Geometry: final body of the model. Coordinates: model frame, mm. A direction names the side the tool comes from. Round coordinates to 2 decimals unless told otherwise and drop trailing zeros. Write each loop counter-clockwise with the first axis right and the second up, starting at its lowest first coordinate (ties: lowest second). Pieces come first, ordered by that corner, then holes. Notation, with made-up numbers: M 52.5,-19.75 L 85.5,-19.75 A21 ccw 85.5,-8.75 Z; hole C 42,31.5 d6. An arc over 180 degrees is marked long. Answer as CSV lines item,"result". Start each with the question number.
Q1. First-contact query: pin 1 (4 mm diameter, centred on y = 25, z = -8, fed in from -X); pin 2 (19.5 mm diameter, centred on x = 14, y = 10, fed in from -Z); pin 3 (19.5 mm diameter, centred on x = 5.5, y = 25.5, fed in from +Z). Flat tips, straight axial feed; report the tip coordinate or a pass-through.
Q2. Ray query, probe 1 along Z at (x, y) = (24, 19.5); probe 2 along X at (y, z) = (25, 31.5); probe 3 along Z at (x, y) = (23.5, 29.5). Return the intervals inside material, ascending.
Q3. Section query D-D on y = 33.5. Output: boundary loops of the cut face in (x, z).
Q4. Section query B-B on z = 17. Output: boundary loops of the cut face in (x, y).
Q5. Section query C-C on x = 0. Output: boundary loops of the cut face in (y, z).
Q6. Mould query, pull axis X, two halves, no side actions, for faces 1 (the flat face through (0, 0, 9)), 2 (the cylindrical face through (5.5, 17.77, -9.87)), 3 (the flat face through (0, 19, 9.206)). Classes: pulls with the +X half, pulls with the -X half, needs draft (parallel to the pull), parting line crosses it, or undercut.
Q7. Reachability of faces 4 (the flat face through (20.554, 19, 20)), 5 (the flat face through (-30.313, 19, 17)) from +Z, -Z, +X, -X, +Y, -Y: full face, straight path, thin tool, end or side. Return the list, or none.
Q8. Section query A-A on y = 19.5. Output: boundary loops of the cut face in (x, z), and give its area (3 significant figures).
```python
from build123d import *

# Parameters (mm, degrees)
F1_DEPTH = 39
F3_R     = 5.308104
F4_DEPTH = 60.626907
F5_R     = 5.76541
F6_DEPTH = 14.8


with BuildPart() as f1:
    # F0 (on Front) → F1 (new body)
    with BuildSketch(Plane.XZ):
        Polygon((0, 9.205531), (0, -2.570523), (30.312954, -2.570523), (30.312954, 36.376152), (20.553786, 36.376152), (20.553786, 9.205531), align=None)
    extrude(amount=-F1_DEPTH)

    # F2: F1 across face


with BuildPart() as f1_1:
    add(f1.part)
    add(f1.part.mirror(Plane(origin=(0, 19.5, 3.317504), x_dir=(0, -1, 0), z_dir=(-1, 0, 0))))

    # F3 (on face) → F4 (cut, through all)
    with BuildSketch(Plane.YZ.offset(30.312954)):
        with Locations((19.5, 27.813217)):
            Circle(F3_R)
    extrude(amount=-F4_DEPTH, mode=Mode.SUBTRACT)

    # F5 (on face) → F6 (join)
    with BuildSketch(Plane(origin=(0, 0, -2.570523), x_dir=(1, 0, 0), z_dir=(0, 0, -1))):
        with Locations((0, -19.5)):
            Circle(F5_R)
    extrude(amount=F6_DEPTH)


solid = f1_1.part
```
Entries:
1,pin 1,"stops at x = -4.58"
1,pin 2,"stops at z = -2.57"
1,pin 3,"stops at z = 9.21"
2,probe 1,"z = -2.57 to 22.51, 33.12 to 36.38"
2,probe 2,"x = -30.31 to -20.55, 20.55 to 30.31"
2,probe 3,"z = -2.57 to 36.38"
3,outline,"M -30.31,-2.57 L 30.31,-2.57 L 30.31,36.38 L 20.55,36.38 L 20.55,9.21 L -20.55,9.21 L -20.55,36.38 L -30.31,36.38 Z"
4,outline,"M -30.31,0 L -20.55,0 L -20.55,39 L -30.31,39 Z; M 20.55,0 L 30.31,0 L 30.31,39 L 20.55,39 Z"
5,outline,"M 0,-2.57 L 13.73,-2.57 L 13.73,-17.37 L 25.27,-17.37 L 25.27,-2.57 L 39,-2.57 L 39,9.21 L 0,9.21 Z"
6,face 1,"needs draft"
6,face 2,"parting line crosses it"
6,face 3,"undercut"
7,face 4,"+Z, +Y, -Y"
7,face 5,"+Z, -Z, -X, +Y, -Y"
8,outline,"M -30.31,-2.57 L -5.77,-2.57 L -5.77,-17.37 L 5.77,-17.37 L 5.77,-2.57 L 30.31,-2.57 L 30.31,22.51 L 20.55,22.51 L 20.55,9.21 L -20.55,9.21 L -20.55,22.51 L -30.31,22.51 Z; M -30.31,33.12 L -20.55,33.12 L -20.55,36.38 L -30.31,36.38 Z; M 20.55,33.12 L 30.31,33.12 L 30.31,36.38 L 20.55,36.38 Z"
8,area,"1,210 mm^2"
